For this review, use the dimensioned drawing (mm, ordinates from the lowest corner) and the shaded views. Coordinates: 2 decimals unless noted, no trailing zeros. Order: outer loops, then holes, each group sorted by start corner. A loop starts at its lowest first (then second) coordinate and runs counter-clockwise, first axis right, second up. Notation, with made-up numbers: M -4.5,67 L 29.5,67 A30 ccw 29.5,95 Z; hole C -13,11 d8. An arc over 180 degrees is marked long. Answer in a Markdown table with one row per item.
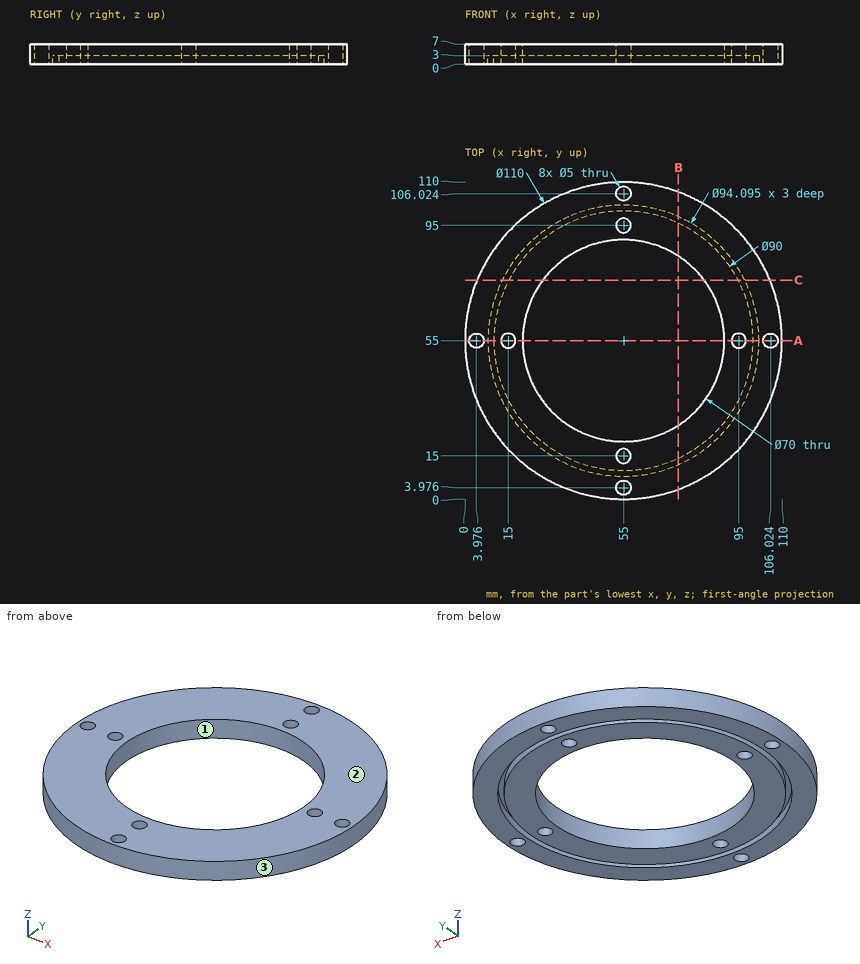
(1) Take a section at A-A (y = 55). State how many separate pieces and enclosed holes the cut face has, then the cut area to 3 significant figures.
Report:
| item | result |
|---|---|
| separate pieces | 6 |
| enclosed holes | 0 |
| area | 128 mm^2 |
(2) The part is to be moulded in two halves that separate along X. For the marked faces 1, 2 and 3, say which applies: +X half, -X half, draft (parallel to the pull), parting line (faces both ways), or undercut.
Report:
| item | result |
|---|---|
| face 1 | undercut |
| face 2 | draft |
| face 3 | parting line |
(3) Insertion check: P1, Ø2, axis at x = 96, y = 52.5, coming from the -Z side; P2, Ø4, axis at x = 55, y = 106.02, coming from the +Z side; P3, Ø2, axis at y = 29, z = 2, coming from the -X side; P4, Ø1.5, axis at y = 26.5, z = 1, coming from the +X side (1 decimal). Each pin has a flat end and moves straight along its axis. Give the tip position at first contact, or say it passes through.
Report:
| item | result |
|---|---|
| P1 | z = 0 |
| P2 | through |
| P3 | x = 6.01 |
| P4 | x = 102.5 |
(4) Take a section at C-C (y = 76). Write out the cut boundary in (x, z), then the cut area to 3 significant figures.
Report:
| item | result |
|---|---|
| outline | M 4.17,0 L 12.9,0 L 12.9,3 L 15.2,3 L 15.2,0 L 27,0 L 27,7 L 4.17,7 Z; M 83,0 L 94.8,0 L 94.8,3 L 97.1,3 L 97.1,0 L 105.83,0 L 105.83,7 L 83,7 Z |
| area | 306 mm^2 |
(5) Take a section at B-B (x = 74). Write out the cut boundary in (y, z).
Report:
| item | result |
|---|---|
| outline | M 3.39,0 L 11.96,0 L 11.96,3 L 14.21,3 L 14.21,0 L 25.61,0 L 25.61,7 L 3.39,7 Z; M 84.39,0 L 95.79,0 L 95.79,3 L 98.04,3 L 98.04,0 L 106.61,0 L 106.61,7 L 84.39,7 Z |
(6) To check wall thickness, follow line 1 (Y direction, x = 55, z = 3.25); line 2 (X direction, y = 67, z = 2) (1 decimal); line 3 (Y direction, x = 91.5, z = 2.5) (1 decimal). State the ranges of each line that lie inside material, in increasing order. Write a range as [from, to].
Report:
| item | result |
|---|---|
| line 1 | [0, 1.48], [6.48, 12.5], [17.5, 20], [90, 92.5], [97.5, 103.52], [108.52, 110] |
| line 2 | [1.3, 9.5], [11.6, 22.1], [87.9, 98.4], [100.5, 108.7] |
| line 3 | [13.9, 25.3], [28.7, 81.3], [84.7, 96.1] |
